```python
from build123d import *

# Parameters (mm, degrees)
SKETCH2_R           = 45
BOSS_EXTRUDE1_DEPTH = 2
SKETCH4_R           = 1.75
CUT_EXTRUDE1_DEPTH  = 64.671029519
SKETCH5_W           = 23
SKETCH5_H           = 12
CUT_EXTRUDE2_DEPTH  = 64.671029519


with BuildPart() as part:
    # Sketch2 → Boss-Extrude1 (new body)
    with BuildSketch(Plane(origin=(0, 0, 0), x_dir=(1, 0, 0), z_dir=(0, 1, 0))):
        with Locations(Location((0, 0, 0), (0, 0, 270))):
            Circle(SKETCH2_R)
    extrude(amount=BOSS_EXTRUDE1_DEPTH)

    # Sketch4 → Cut-Extrude1 (cut, through all)
    with BuildSketch(Plane(origin=(0, 2, 0), x_dir=(1, 0, 0), z_dir=(0, 1, 0))):
        with Locations(Location((0, 40, 0), (0, 0, 270))):
            Circle(SKETCH4_R)
        with Locations(Location((40, 0, 0), (0, 0, 270))):
            Circle(SKETCH4_R)
        with Locations(Location((0, -40, 0), (0, 0, 270))):
            Circle(SKETCH4_R)
        with Locations(Location((-40, 0, 0), (0, 0, 270))):
            Circle(SKETCH4_R)
    extrude(amount=-CUT_EXTRUDE1_DEPTH, mode=Mode.SUBTRACT)

    # Sketch5 → Cut-Extrude2 (cut, through all)
    with BuildSketch(Plane.XZ):
        Rectangle(SKETCH5_W, SKETCH5_H)
    extrude(amount=-CUT_EXTRUDE2_DEPTH, mode=Mode.SUBTRACT)


solid = part.part
```
For this review, take the finished solid that the model builds, in its own axes (mm). A direction names the side the tool comes from. Give positions to 0.01 mm unless a question says otherwise; leave off trailing zeros. Write each loop counter-clockwise with the first axis right and the second up, starting at its lowest first coordinate (ties: lowest second). Pieces come first, ordered by that corner, then holes.
Item 1: Take a section at C-C (x = 0). Give the boundary of the cut face in (y, z), and give its area (3 significant figures).
Item 2: Machinability: for faces 1 (the face through (1, 2, 9)), 2 (the face through (0, 1, 6)), which of the approach directions +Z, -Z, +X, -X, +Y, -Y give a long, thin tool a straight path to every point of the face, cutting with its end or side? Answer none if there is none.
Item 3: Wall thickness on probe 1 along X at (y, z) = (1, 0); probe 2 along Z at (x, y) = (-9, 1.65); probe 3 along X at (y, z) = (1.2, 41.5): over which ranges is each line inside the solid? List them lowest first.
Item 4: Insertion check: P1, Ø1, axis at y = 0.5, z = 34.5, coming from the -X side; P2, Ø1, axis at y = 1.5, z = -1.5, coming from the +X side; P3, Ø2, axis at x = -1.5, z = -3.5, coming from the -Y side; P4, Ø1, axis at x = 3.5, y = 1.5, coming from the +Z side. Each pin has a flat end and moves straight along its axis. Give the tip position at first contact, or say it passes through.
Item 5: Take a section at A-A (z = 0). Give the boundary of the cut face in (x, y), and give its area (3 significant figures).
Item 6: Take a section at D-D (z = -40). Give the boundary of the cut face in (x, y).
Item 7: Take a section at B-B (y = 1.7). Give the boundary of the cut face in (x, z), and give its area (3 significant figures).
Item 8: The part is to be moulded in two halves that separate along X. For faces 3 (the face through (-41.71, 1.01, -0.38)), 4 (the face through (11.5, 1, 0)), 5 (the face through (1, 0, 9)), 6 (the face through (-17.235, 0.986, 41.569)), say which applies: +X half, -X half, draft (parallel to the pull), parting line (faces both ways), or undercut.
Established:
1. outline: (0, -45) - (2, -45) - (2, -41.75) - (0, -41.75) - close; (0, -38.25) - (2, -38.25) - (2, -6) - (0, -6) - close; (0, 6) - (2, 6) - (2, 38.25) - (0, 38.25) - close; (0, 41.75) - (2, 41.75) - (2, 45) - (0, 45) - close
1. area: 142 mm2
2. face 1: +Z, -Z, +X, -X, +Y
2. face 2: +Y, -Y
3. probe 1: x = -45 to -41.75, -38.25 to -11.5, 11.5 to 38.25, 41.75 to 45
3. probe 2: z = -44.09 to -6, 6 to 44.09
3. probe 3: x = -17.4 to -0.9, 0.9 to 17.4
4. P1: stops at x = -29.48
4. P2: stops at x = 44.99
4. P3: passes through
4. P4: stops at z = 44.9
5. outline: (-45, 0) - (-41.75, 0) - (-41.75, 2) - (-45, 2) - close; (-38.25, 0) - (-11.5, 0) - (-11.5, 2) - (-38.25, 2) - close; (11.5, 0) - (38.25, 0) - (38.25, 2) - (11.5, 2) - close; (41.75, 0) - (45, 0) - (45, 2) - (41.75, 2) - close
5. area: 120 mm2
6. outline: (-20.62, 0) - (-1.75, 0) - (-1.75, 2) - (-20.62, 2) - close; (1.75, 0) - (20.62, 0) - (20.62, 2) - (1.75, 2) - close
7. outline: circle Ø90 at (0, 0); hole circle Ø3.5 at (-40, 0); hole (-11.5, -6) - (11.5, -6) - (11.5, 6) - (-11.5, 6) - close; hole circle Ø3.5 at (0, -40); hole circle Ø3.5 at (0, 40); hole circle Ø3.5 at (40, 0)
7. area: 6,050 mm2
8. face 3: undercut
8. face 4: undercut
8. face 5: draft
8. face 6: parting line
